Design review of the part built by this model. Coordinates are the model's own, in mm. Coordinates: 2 decimals unless noted, no trailing zeros. Loops run counter-clockwise (first coordinate to the right, second up) from the corner with the lowest first, then second, coordinate; pieces in that order, holes last. Notation, with made-up numbers: M 77,56.5 L 112,56.5 A29 cw 112,95.5 Z; hole C 72.5,65 d11. An arc over 180 degrees is marked long. Write item = value, one per line. Start each with the question number.
Autodesk Inventor part; units mm, degrees
ref_plane "YZ Plane" through (0, 0, 0) normal (1, 0, 0) x (0, 1, 0)
ref_plane "XZ Plane" through (0, 0, 0) normal (0, 1, 0) x (-1, 0, 0)
ref_plane "XY Plane" through (0, 0, 0) normal (0, 0, 1) x (1, 0, 0)
sketch "スケッチ1" plane through (0, 0, 0) normal (0, 0, 1) x (1, 0, 0)
  circle A0 centre (0, 0) radius 4
  circle A1 centre (0, 0) radius 8
  circle A2 centre (0, 0) radius 6 construction
  circle A3 centre (0, 6) radius 1.1
  circle A4 centre (-4.2426, 4.2426) radius 1.1
  circle A5 centre (-6, 0) radius 1.1
  circle A6 centre (-4.2426, -4.2426) radius 1.1
  circle A7 centre (0, -6) radius 1.1
  circle A8 centre (4.2426, -4.2426) radius 1.1
  circle A9 centre (6, 0) radius 1.1
  circle A10 centre (4.2426, 4.2426) radius 1.1
  arc A11 (8.483, -10.1137) -> (9.4351, -9.068) centre (8.4362, -9.1148) ccw
  circle A12 centre (0, 0) radius 13.4197 construction
  circle A13 centre (0, 0) radius 19.4197 construction
  line L0 (5, -19.4197) -> (-5, -19.4197)
  line L1 (-5, -19.4197) -> (-5, -22.4197)
  line L2 (-5, -22.4197) -> (5, -22.4197)
  line L3 (5, -22.4197) -> (5, -19.4197)
  circle A14 centre (3.9, -19.4197) radius 1.1
  line L4 (0, -19.4197) -> (0, -22.4197) construction
  line L5 (0, -20.9197) -> (5, -20.9197) construction
  circle A15 centre (3.9, -22.4197) radius 1.1
  circle A16 centre (-3.9, -19.4197) radius 1.1
  circle A17 centre (-3.9, -22.4197) radius 1.1
  circle A18 centre (10, -20.9197) radius 1.1
  circle A19 centre (-10, -20.9197) radius 1.1
  circle A20 centre (10, -20.9197) radius 2
  circle A21 centre (-10, -20.9197) radius 2
  line L6 (11.9662, -20.5535) -> (7.8647, 1.465)
  line L7 (-11.9662, -20.5535) -> (-7.8647, 1.465)
  circle A22 centre (3.9, -22.4197) radius 2
  circle A23 centre (-3.9, -22.4197) radius 2
  line L8 (3.9, -24.4197) -> (-3.9, -24.4197)
  line L9 (-3.9, -24.4197) -> (-10.4609, -22.8659)
  line L10 (3.9, -24.4197) -> (10.4609, -22.8659)
  point P0 (-5, -19.4197)
  point P1 (-2.8, -19.4197)
  point P2 (2.8, -19.4197)
  point P3 (5, -22.4197)
  point P4 (2.8, -22.4197)
  point P5 (-5, -22.4197)
  point P6 (-5, -22.4197)
  point P7 (-7.8647, 1.465)
  point P8 (-11.9662, -20.5535)
  point P9 (-2.8, -22.4197)
  dimension "d1" = 16
  dimension "d2" = 12
  dimension "d13" = 2.2
  dimension "d17" = 4
  dimension "d18" = 4
  dimension "d19" = 4
  dimension "d0" = 8
  dimension "d3" = 2.2
  dimension "d6" = 360
  dimension "d10" = 6
  dimension "d11" = 10
  dimension "d12" = 3
  dimension "d14" = 2.2
  dimension "d15" = 5
  dimension "d16" = 4
extrude "押し出し1" add sketch "スケッチ1" along normal blind 1.5 contours A1 | A1 L6 A20 L10 A22 L3 A14 L0 A16 L1 A23 L9 A21 L7 | A20 | A21 | L10 A22 L2 A15 L3 | A23 L1 A17 L2 L9 | L8 A23 L2 A22
sketch "スケッチ2" plane through (0, 0, 0) normal (0, 0, -1) x (-1, 0, 0)
  circle A0 centre (0, 0) radius 8
  arc A1 (7.8647, 1.465) -> (-7.8647, 1.465) centre (0, 0) ccw
  line L0 (-8.1259, -16.3197) -> (8.1259, -16.3197)
  line L1 (8.1259, -16.3197) -> (6.0591, -5.2238)
  line L2 (-6.0591, -5.2238) -> (-8.1259, -16.3197)
  line L3 (7.8647, 1.465) -> (11.9662, -20.5535)
  line L4 (-11.9662, -20.5535) -> (-7.8647, 1.465)
  arc A2 (-2.8, -19.4197) -> (-5, -19.4197) centre (-3.9, -19.4197) ccw
  point P0 (9.9154, -9.5443)
  point P1 (-3.9, -18.3197)
  dimension "d20" = 3
  dimension "d21" = 3
  dimension "d22" = 2
extrude "押し出し2" cut sketch "スケッチ2" against normal through all contours L1 L0 L2 A0
fillet "フィレット1" radius 2 4 edges at (6.0591, -5.2238, 0.75) (-6.0591, -5.2238, 0.75) (-8.1259, -16.3197, 0.75) (8.1259, -16.3197, 0.75)
equation "\"d21\" = d20"
properties part number "mataroll" material "アルミニウム 2014-T4"
(1) Mouldability with a two-part tool opening along Y and no side actions: class faces 1 (the cylindrical face through (0, 8, 1)), 2 (the flat face through (-7.135, -23.654, 0.74)), 3 (the cylindrical face through (-4.984, 0.421, 0.74)), 4 (the cylindrical face through (4.75, -3.267, 0.74)) as +Y half, -Y half, draft (parallel to the pull), parting line (faces both ways), or undercut.
(2) Take a section at A-A (x = 0.5). State the section outline as (y, z) points, plus the area to 3 significant figures.
(3) To check wall thickness, follow L1, parallel to Y at x = 0, z = 1.25; L2, parallel to Y at x = 4.5, z = 0.45; L3, parallel to X at y = -1, z = 1.2. State the ranges of each line that lie inside material, in increasing order.
(4) Take a section at C-C (x = 10). State the section outline as (y, z) points.
(5) Take a section at D-D (z = 0.9). Give the number of separate pieces and of enclosed holes in the cut face, plus the area to 3 significant figures.
(6) Insertion check: pin 1 (1.8 mm diameter, centred on x = -10, y = -20.92, fed in from -Z); pin 2 (3 mm diameter, centred on x = 0, y = -6, fed in from +Z). Each pin has a flat end and moves straight along its axis. Give the tip position at first contact, or say it passes through.
(7) Take a section at B-B (y = -2). State the section outline as (x, z) points, plus the area to 3 significant figures.
Results list:
q1.face_1 = +Y half
q1.face_2 = -Y half
q1.face_3 = undercut
q1.face_4 = undercut
q2.outline = M -24.42,0 L -22.42,0 L -22.42,1.5 L -24.42,1.5 Z; M -19.42,0 L -16.32,0 L -16.32,1.5 L -19.42,1.5 Z; M -7.98,0 L -6.98,0 L -6.98,1.5 L -7.98,1.5 Z; M -5.02,0 L -3.97,0 L -3.97,1.5 L -5.02,1.5 Z; M 3.97,0 L 5.02,0 L 5.02,1.5 L 3.97,1.5 Z; M 6.98,0 L 7.98,0 L 7.98,1.5 L 6.98,1.5 Z
q2.area = 13.8 mm^2
q3.L1 = -24.42 to -22.42, -19.42 to -16.32, -8 to -7.1, -4.9 to -4, 4 to 4.9, 7.1 to 8
q3.L2 = -24.28 to -23.34, -18.5 to -16.32, -6.84 to -5.31, -3.17 to 3.17, 5.31 to 6.61
q3.L3 = -8.32 to -6.46, -5.54 to -3.87, 3.87 to 5.54, 6.46 to 8.32
q4.outline = M -22.98,0 L -22.02,0 L -22.02,1.5 L -22.98,1.5 Z; M -19.82,0 L -10,0 L -10,1.5 L -19.82,1.5 Z
q5.separate_pieces = 1
q5.enclosed_holes = 13
q5.area = 337 mm^2
q6.pin_1 = through
q6.pin_2 = 1.5
q7.outline = M -8.51,0 L -3.46,0 L -3.46,1.5 L -8.51,1.5 Z; M 3.46,0 L 8.51,0 L 8.51,1.5 L 3.46,1.5 Z
q7.area = 15.1 mm^2
